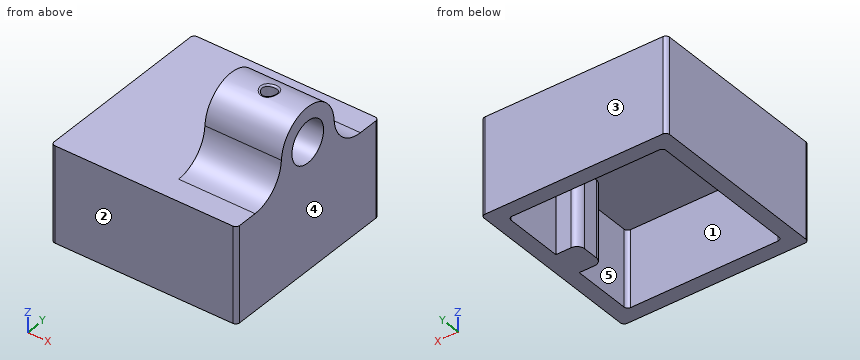
from build123d import *

# Parameters (mm, degrees)
SKETCH2_W           = 4
SKETCH2_H           = 8
SKETCH2_W_2         = 6
BOSS_EXTRUDE1_DEPTH = 5
SKETCH3_R           = 5.4
BOSS_EXTRUDE2_DEPTH = 10
SKETCH2_3_W         = 6
SKETCH2_3_H         = 8
SKETCH2_3_W_2       = 4
BOSS_EXTRUDE3_DEPTH = 20
FILLET1_R           = 2
SKETCH4_R           = 1.9
CUT_EXTRUDE1_DEPTH  = 10
FILLET2_R           = 0.4


with BuildPart() as part:
    # Sketch2 → Boss-Extrude1 (new body)
    with BuildSketch(Plane.XY):
        with BuildLine():
            Line((14.25, 4), (20.25, 4))
            Line((20.25, 4), (20.25, 19.25))
            ThreePointArc((20.25, 19.25), (19.957106781, 19.957106781), (19.25, 20.25))
            Line((19.25, 20.25), (-19.25, 20.25))
            ThreePointArc((-19.25, 20.25), (-19.957106781, 19.957106781), (-20.25, 19.25))
            Line((-20.25, 19.25), (-20.25, -19.25))
            ThreePointArc((-20.25, -19.25), (-19.957106781, -19.957106781), (-19.25, -20.25))
            Line((-19.25, -20.25), (19.25, -20.25))
            ThreePointArc((19.25, -20.25), (19.957106781, -19.957106781), (20.25, -19.25))
            Line((20.25, -19.25), (20.25, -4))
            Line((20.25, -4), (14.25, -4))
            Line((14.25, -4), (14.25, 4))
        make_face()
        with BuildLine():
            Line((23.25, 24.25), (-23.25, 24.25))
            ThreePointArc((-23.25, 24.25), (-23.957106781, 23.957106781), (-24.25, 23.25))
            Line((-24.25, 23.25), (-24.25, -23.25))
            ThreePointArc((-24.25, -23.25), (-23.957106781, -23.957106781), (-23.25, -24.25))
            Line((-23.25, -24.25), (23.25, -24.25))
            ThreePointArc((23.25, -24.25), (23.957106781, -23.957106781), (24.25, -23.25))
            Line((24.25, -23.25), (24.25, -4))
            Line((24.25, -4), (20.25, -4))
            Line((20.25, -4), (20.25, -19.25))
            ThreePointArc((20.25, -19.25), (19.957106781, -19.957106781), (19.25, -20.25))
            Line((19.25, -20.25), (-19.25, -20.25))
            ThreePointArc((-19.25, -20.25), (-19.957106781, -19.957106781), (-20.25, -19.25))
            Line((-20.25, -19.25), (-20.25, 19.25))
            ThreePointArc((-20.25, 19.25), (-19.957106781, 19.957106781), (-19.25, 20.25))
            Line((-19.25, 20.25), (19.25, 20.25))
            ThreePointArc((19.25, 20.25), (19.957106781, 19.957106781), (20.25, 19.25))
            Line((20.25, 19.25), (20.25, 4))
            Line((20.25, 4), (24.25, 4))
            Line((24.25, 4), (24.25, 23.25))
            ThreePointArc((24.25, 23.25), (23.957106781, 23.957106781), (23.25, 24.25))
        make_face()
        with Locations((22.25, 0)):
            Rectangle(SKETCH2_W, SKETCH2_H)
        with Locations((17.25, 0)):
            Rectangle(SKETCH2_W_2, SKETCH2_H)
    extrude(amount=BOSS_EXTRUDE1_DEPTH)

    # Sketch3 → Boss-Extrude2 (add, symmetric)
    with BuildSketch(Plane(origin=(14.25, 0, 0), x_dir=(0, 0, -1), z_dir=(1, 0, 0))):
        with BuildLine():
            Line((-5, -17.972200756), (-5, 17.972200756))
            ThreePointArc((-5, 17.972200756), (-7.461651585, 11.787542317), (-13.5, 8.986100378))
            ThreePointArc((-13.5, 8.986100378), (-22, 0), (-13.5, -8.986100378))
            ThreePointArc((-13.5, -8.986100378), (-7.461651585, -11.787542317), (-5, -17.972200756))
        make_face()
        with Locations((-13, 0)):
            Circle(SKETCH3_R, mode=Mode.SUBTRACT)
    extrude(amount=BOSS_EXTRUDE2_DEPTH, both=True)

    # Sketch2_3 → Boss-Extrude3 (add)
    with BuildSketch(Plane.XY):
        with Locations((17.25, 0)):
            Rectangle(SKETCH2_3_W, SKETCH2_3_H)
        with BuildLine():
            Line((23.25, 24.25), (-23.25, 24.25))
            ThreePointArc((-23.25, 24.25), (-23.957106781, 23.957106781), (-24.25, 23.25))
            Line((-24.25, 23.25), (-24.25, -23.25))
            ThreePointArc((-24.25, -23.25), (-23.957106781, -23.957106781), (-23.25, -24.25))
            Line((-23.25, -24.25), (23.25, -24.25))
            ThreePointArc((23.25, -24.25), (23.957106781, -23.957106781), (24.25, -23.25))
            Line((24.25, -23.25), (24.25, -4))
            Line((24.25, -4), (20.25, -4))
            Line((20.25, -4), (20.25, -19.25))
            ThreePointArc((20.25, -19.25), (19.957106781, -19.957106781), (19.25, -20.25))
            Line((19.25, -20.25), (-19.25, -20.25))
            ThreePointArc((-19.25, -20.25), (-19.957106781, -19.957106781), (-20.25, -19.25))
            Line((-20.25, -19.25), (-20.25, 19.25))
            ThreePointArc((-20.25, 19.25), (-19.957106781, 19.957106781), (-19.25, 20.25))
            Line((-19.25, 20.25), (19.25, 20.25))
            ThreePointArc((19.25, 20.25), (19.957106781, 19.957106781), (20.25, 19.25))
            Line((20.25, 19.25), (20.25, 4))
            Line((20.25, 4), (24.25, 4))
            Line((24.25, 4), (24.25, 23.25))
            ThreePointArc((24.25, 23.25), (23.957106781, 23.957106781), (23.25, 24.25))
        make_face()
        with Locations((22.25, 0)):
            Rectangle(SKETCH2_3_W_2, SKETCH2_3_H)
    extrude(amount=-BOSS_EXTRUDE3_DEPTH)

    # Fillet1
    fillet1_edges = [part.edges().sort_by_distance(p)[0] for p in [
        (14.25, -4, -10),
        (14.25, 4, -10),
    ]]
    fillet(fillet1_edges, radius=FILLET1_R)

    # Sketch4 → Cut-Extrude1 (cut)
    with BuildSketch(Plane.XY.offset(22)):
        with Locations((14.25, 0)):
            Circle(SKETCH4_R)
    extrude(amount=-CUT_EXTRUDE1_DEPTH, mode=Mode.SUBTRACT)

    # Fillet2
    fillet2_edges = [part.edges().sort_by_distance(p)[0] for p in [
        (12.349999989, 0, 21.999999997),
    ]]
    fillet(fillet2_edges, radius=FILLET2_R)


solid = part.part
Could you check a few things on this model? Use its own coordinates, in mm. Face numbers are marked on the shaded views. A direction names the side the tool comes from. Coordinates: 2 decimals unless noted, no trailing zeros. Write each loop counter-clockwise with the first axis right and the second up, starting at its lowest first coordinate (ties: lowest second). Pieces come first, ordered by that corner, then holes. Notation, with made-up numbers: M -28.75,59 L 30.25,59 A11 ccw 30.25,67 Z; hole C -13,20 d5. An arc over 180 degrees is marked long. One line per question, with ' | ' between items.
1) Imagine slicing it at C-C, the plane z = 14.5. Write out the boundary of the cut face in (x, y), and give its area (3 significant figures).
Checks:
outline: M 4.25,-8.87 L 24.25,-8.87 L 24.25,-5.19 L 4.25,-5.19 Z; M 4.25,5.19 L 24.25,5.19 L 24.25,8.87 L 4.25,8.87 Z | area: 147 mm²
2) Imagine slicing it at A-A, the plane x = 21. Write out the boundary of the cut face in (y, z).
Checks:
outline: M -24.25,-20 L 24.25,-20 L 24.25,5 L 17.97,5 A9 cw 8.99,13.5 A9 ccw -8.99,13.5 A9 cw -17.97,5 L -24.25,5 Z; hole C 0,13 d10.8
3) I need wall thicknesses on probe 1 along Y at (x, z) = (16, -14); probe 2 along Y at (x, z) = (2.5, -8). Which ranges of each line are inside material? Lowest first, please. Write a range as [from, to].
Checks:
probe 1: [-24.25, -20.25], [-3.98, 3.98], [20.25, 24.25] | probe 2: [-24.25, -20.25], [20.25, 24.25]
4) If we mould it in two halves opening along X, with no side actions, what happens to the marked faces 3, 4 and 5? For each: released by +X, released by -X, zero draft, split by the parting line, or undercut.
Checks:
face 3: zero draft | face 4: released by +X | face 5: undercut
5) For pin 1 Ø14.5 at (x, y) = (-8, -0.5) entering from +Z; pin 2 Ø6 at (x, y) = (-8, -12.5) entering from -Z; pin 3 Ø10 at (x, y) = (3, 5) entering from +Z, each with a flat end and sliding along its axis, tell me the tip position at first contact or that it passes through.
Checks:
pin 1: z = 5 | pin 2: z = 0 | pin 3: z = 22
6) For the marked faces 1 and 2, which set-ups out of +Z, -Z, +X, -X, +Y, -Y let a thin tool reach every point of the face, with its end or its side?
Checks:
face 1: -Z | face 2: +Z, -Z, +X, -X, -Y
7) Imagine slicing it at B-B, the plane y = 0. Give the number of separate pieces and of enclosed holes in the cut face, and give its area (3 significant figures).
Checks:
separate pieces: 3 | enclosed holes: 0 | area: 633 mm²
8) Imagine slicing it at D-D, the plane x = 5. Write out the boundary of the cut face in (y, z).
Checks:
outline: M -24.25,-20 L -20.25,-20 L -20.25,0 L 20.25,0 L 20.25,-20 L 24.25,-20 L 24.25,5 L 17.97,5 A9 cw 8.99,13.5 A9 ccw -8.99,13.5 A9 cw -17.97,5 L -24.25,5 Z; hole C 0,13 d10.8
